Here's the drawing with two shaded views (mm, measured from the low corner). I have some questions. Round coordinates to 2 decimals unless told otherwise and drop trailing zeros. Order: outer loops, then holes, each group sorted by start corner. A loop starts at its lowest first (then second) coordinate and runs counter-clockwise, first axis right, second up.
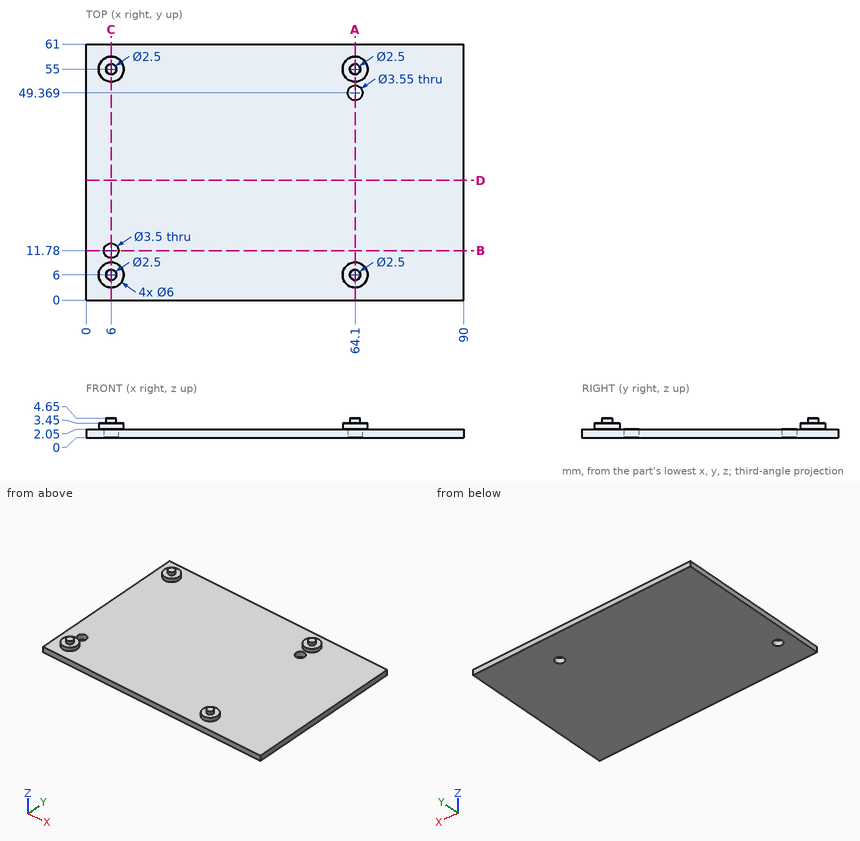
1. If we section it at A-A, the plane x = 64.1: Write out the boundary of the cut face in (y, z).
Evaluation:
outline: (0, 0) - (47.59, 0) - (47.59, 2.05) - (9, 2.05) - (9, 3.45) - (7.25, 3.45) - (7.25, 4.65) - (4.75, 4.65) - (4.75, 3.45) - (3, 3.45) - (3, 2.05) - (0, 2.05) - close; (51.14, 0) - (61, 0) - (61, 2.05) - (58, 2.05) - (58, 3.45) - (56.25, 3.45) - (56.25, 4.65) - (53.75, 4.65) - (53.75, 3.45) - (52, 3.45) - (52, 2.05) - (51.14, 2.05) - close
2. I need wall thicknesses on probe 1 along Y at (x, z) = (6, 1.05); probe 2 along Y at (x, z) = (64.1, 1.45); probe 3 along Z at (x, y) = (15, 44). Which ranges of each line are inside material? Lowest first, please.
Evaluation:
probe 1: y = 0 to 10.03, 13.53 to 61
probe 2: y = 0 to 47.59, 51.14 to 61
probe 3: z = 0 to 2.05
3. If we section it at B-B, the plane y = 11.78: Write out the boundary of the cut face in (x, z), and give its area (3 significant figures).
Evaluation:
outline: (0, 0) - (4.25, 0) - (4.25, 2.05) - (0, 2.05) - close; (7.75, 0) - (90, 0) - (90, 2.05) - (7.75, 2.05) - close
area: 177 mm2
4. I'm going to push a flat-ended pin straight in: P1, Ø1.8, axis at x = 7.5, y = 6.5, coming from the +Z side. Where does the tip first touch, or does it pass through?
Evaluation:
P1: stops at z = 4.65
5. If we section it at C-C, the plane x = 6: Write out the boundary of the cut face in (y, z).
Evaluation:
outline: (0, 0) - (10.03, 0) - (10.03, 2.05) - (9, 2.05) - (9, 3.45) - (7.25, 3.45) - (7.25, 4.65) - (4.75, 4.65) - (4.75, 3.45) - (3, 3.45) - (3, 2.05) - (0, 2.05) - close; (13.53, 0) - (61, 0) - (61, 2.05) - (58, 2.05) - (58, 3.45) - (56.25, 3.45) - (56.25, 4.65) - (53.75, 4.65) - (53.75, 3.45) - (52, 3.45) - (52, 2.05) - (13.53, 2.05) - close
6. If we section it at D-D, the plane y = 28.5: Write out the boundary of the cut face in (x, z).
Evaluation:
outline: (0, 0) - (90, 0) - (90, 2.05) - (0, 2.05) - close
